```python
from build123d import *
from build123d.topology import SkipClean

# Parameters (mm, degrees)
EXTRUDE_1_DEPTH          = 80
SKETCH_2_R               = 13
CUT_EXTRUDE_2_DEPTH      = 15
CUT_EXTRUDE_START        = -15
SKETCH_4_R               = 13
CUT_EXTRUDE_3_DEPTH      = 15
CUT_EXTRUDE_4_DEPTH      = 123.918354375
CUT_EXTRUDE_4_DEPTH_BACK = 123.918354375
SKETCH_5_W               = 20
SKETCH_5_H               = 40
CUT_EXTRUDE_6_DEPTH      = 123.918354375
CUT_EXTRUDE_6_DEPTH_BACK = 24
CUT_EXTRUDE_7_DEPTH      = 131.345394404
CUT_EXTRUDE_8_DEPTH      = 32
CUT_EXTRUDE_8_DEPTH_BACK = 24
SKETCH_10_W              = 30
SKETCH_10_H              = 40
CUT_EXTRUDE_9_DEPTH      = 6
SKETCH_13_W              = 10.619852086
SKETCH_13_H              = 40
CUT_EXTRUDE_10_DEPTH     = 71
EXTRUDE_3_DEPTH          = 60


with BuildPart() as part:
    # Эскиз1 → Бобышка-Вытянуть1 (new body)
    with BuildSketch(Plane.XY):
        with BuildLine():
            Line((-84.314422505, -30), (-23.694570419, 25.759800711))
            ThreePointArc((-23.694570419, 25.759800711), (28.113366731, 20.847988178), (17.769230769, -30.153846154))
            Line((17.769230769, -30.153846154), (1.060606061, -40))
            Line((1.060606061, -40), (-84.314422505, -40))
            Line((-84.314422505, -40), (-84.314422505, -30))
        make_face()
    extrude(amount=EXTRUDE_1_DEPTH)

    # Эскиз2 → Вырез-Вытянуть2 (cut)
    with BuildSketch(Plane.XY):
        Circle(SKETCH_2_R)
    extrude(amount=CUT_EXTRUDE_2_DEPTH, mode=Mode.SUBTRACT)

    # Эскиз4 → Вырез-Вытянуть3 (cut)
    with BuildSketch(Plane.XY.offset(80).offset(CUT_EXTRUDE_START)):
        Circle(SKETCH_4_R)
    extrude(amount=CUT_EXTRUDE_3_DEPTH, mode=Mode.SUBTRACT)

    # Эскиз5 → Вырез-Вытянуть4 (cut, two sides: drawn at the far end of the back side and taken through both)
    with BuildSketch(Plane(origin=(0, 0, 0), x_dir=(1, 0, 0), z_dir=(0, 1, 0)).offset(-CUT_EXTRUDE_4_DEPTH_BACK)):
        with Locations((-74.314422505, -40)):
            Rectangle(SKETCH_5_W, SKETCH_5_H)
    extrude(amount=CUT_EXTRUDE_4_DEPTH + CUT_EXTRUDE_4_DEPTH_BACK, mode=Mode.SUBTRACT)

    # Эскиз6 → Вырез-Вытянуть6 (cut, two sides: drawn at the far end of the back side and taken through both)
    with BuildSketch(Plane(origin=(0, 0, 0), x_dir=(1, 0, 0), z_dir=(0, 1, 0)).offset(-CUT_EXTRUDE_6_DEPTH_BACK)):
        with BuildLine():
            Line((-55, -25), (-84.314422505, -25))
            Line((-84.314422505, -25), (-84.314422505, -55))
            Line((-84.314422505, -55), (-55, -55))
            ThreePointArc((-55, -55), (-40, -40), (-55, -25))
        make_face()
    extrude(amount=CUT_EXTRUDE_6_DEPTH + CUT_EXTRUDE_6_DEPTH_BACK, mode=Mode.SUBTRACT)

    # Эскиз9 → Вырез-Вытянуть7 (cut, through all)
    with BuildSketch(Plane(origin=(0, -24, 0), x_dir=(1, 0, 0), z_dir=(0, 1, 0))):
        with BuildLine():
            Line((-55, -48), (-92.733432528, -48))
            Line((-92.733432528, -48), (-92.733432528, -32))
            Line((-92.733432528, -32), (-55, -32))
            ThreePointArc((-55, -32), (-47, -40), (-55, -48))
        make_face()
    extrude(amount=-CUT_EXTRUDE_7_DEPTH, mode=Mode.SUBTRACT)

    # Эскиз10 → Вырез-Вытянуть8 (cut, two sides: drawn at the far end of the back side and taken through both)
    with BuildSketch(Plane(origin=(0, 0, 0), x_dir=(1, 0, 0), z_dir=(0, 1, 0)).offset(-CUT_EXTRUDE_8_DEPTH_BACK)):
        with Locations((-49.314422505, -40)):
            Rectangle(SKETCH_10_W, SKETCH_10_H)
    extrude(amount=CUT_EXTRUDE_8_DEPTH + CUT_EXTRUDE_8_DEPTH_BACK, mode=Mode.SUBTRACT)

    # Эскиз11 → Вырез-Вытянуть9 (cut)
    with BuildSketch(Plane(origin=(0, -24, 0), x_dir=(1, 0, 0), z_dir=(0, 1, 0))):
        with BuildLine():
            Line((-55, -25), (-81.861005174, -25))
            Line((-81.861005174, -25), (-81.861005174, -55))
            Line((-81.861005174, -55), (-55, -55))
            ThreePointArc((-55, -55), (-40, -40), (-55, -25))
        make_face()
    extrude(amount=-CUT_EXTRUDE_9_DEPTH, mode=Mode.SUBTRACT)

    # Эскиз13 → Вырез-Вытянуть10 (cut)
    with BuildSketch(Plane(origin=(0, -24, 0), x_dir=(1, 0, 0), z_dir=(0, 1, 0))):
        with Locations((-29.004496462, -40)):
            Rectangle(SKETCH_13_W, SKETCH_13_H)
    extrude(amount=CUT_EXTRUDE_10_DEPTH, mode=Mode.SUBTRACT)

    # Эскиз12 → Бобышка-Вытянуть3 (add)
    with SkipClean():  # the faces are left unmerged after this step: merging them gives an invalid solid
        with BuildSketch(Plane.XY):
            with BuildLine():
                Line((-35, 0), (-35, -24))
                Line((-35, -24), (-25.475478406, -24))
                ThreePointArc((-25.475478406, -24), (32.53184397, 12.9104271), (-35, 0))
            make_face()
        extrude(amount=EXTRUDE_3_DEPTH)


solid = part.part
```
Check sheet for the modelled part. Datum: model origin and axes. Units: mm. A direction names the side the tool comes from. Coordinates: 2 decimals unless noted, no trailing zeros. Order: outer loops, then holes, each group sorted by start corner. A loop starts at its lowest first (then second) coordinate and runs counter-clockwise, first axis right, second up. Notation, with made-up numbers: (34, 29.5) -> (62, 29.5) arc R34 cw to (62, 65.5) -> close; hole circle Ø6 at (73, 30). An arc over 180 degrees is marked (long way). Write each question's results on one line, items separated by ' | '. Start each with the question number.
1) Material ranges on line 1 along Z through (x, y) = (-50, -2); line 2 along Y through (x, z) = (0, 75.5); line 3 along Z through (x, y) = (5.5, -5), recorded low to high.
2) Section check D-D (z = 40). Enter the section's corners in (x, y).
3) Draft check along Z on faces 4 (the face through (-10.316, -7.91, 72.395)), 5 (the face through (0, 0, 65)), 6 (the face through (-60, -27, 25)), 7 (the face through (-60, -35, 32)). Enter one of: pulls with the +Z half, pulls with the -Z half, needs draft (parallel to the pull), parting line crosses it, or undercut.
4) Depth check by flat-ended pin: pin 1 (1.5 mm diameter, centred on y = -16, z = 63.5, fed in from -X); pin 2 (7 mm diameter, centred on y = -11.5, z = 38, fed in from -X); pin 3 (3.5 mm diameter, centred on y = -29.5, z = 56.5, fed in from -X). Enter the tip coordinate at first touch or a pass-through.
5) Section check C-C (y = 9). Enter the section's corners in (x, z), and give its area (3 significant figures).
6) Section check A-A (z = 67). Enter the section's corners in (x, y).
7) Section check B-B (x = -57.5). Enter the section's corners in (y, z), and give its area (3 significant figures).
8) Set-up check for faces 1 (the face through (-11, -10, 80)), 2 (the face through (-40, -27, 40)), 3 (the face through (-60, -35, 48)): record each of +Z, -Z, +X, -X, +Y, -Y from which the full face is reachable in a straight line by a thin tool's end or side.
Checked values:
1) line 1: 0 to 20, 60 to 80 | line 2: -40 to -13, 13 to 35 | line 3: 0 to 65
2) outline: (-47, -40) -> (1.06, -40) -> (17.77, -30.15) arc R35 ccw (long way) to (-35, 0) -> (-35, -24) -> (-40, -24) -> (-40, -30) -> (-47, -30) -> close
3) face 4: needs draft | face 5: pulls with the +Z half | face 6: undercut | face 7: undercut
4) pin 1: x = -69.91 | pin 2: x = -35 | pin 3: x = -64.31
5) outline: (-41.92, 0) -> (33.82, 0) -> (33.82, 80) -> (9.38, 80) -> (9.38, 65) -> (-9.38, 65) -> (-9.38, 80) -> (-41.92, 80) -> (-41.92, 60) -> (-33.82, 60) -> (-33.82, 20) -> (-41.92, 20) -> close | area: 5,450 mm²
6) outline: (-84.31, -40) -> (1.06, -40) -> (17.77, -30.15) arc R35 ccw (long way) to (-23.69, 25.76) -> (-84.31, -30) -> close; hole circle Ø26 at (0, 0)
7) outline: (-40, 0) -> (-5.34, 0) -> (-5.34, 20) -> (-24, 20) -> (-24, 25) -> (-30, 25) -> (-30, 32) -> (-40, 32) -> close; (-40, 48) -> (-30, 48) -> (-30, 55) -> (-24, 55) -> (-24, 60) -> (-5.34, 60) -> (-5.34, 80) -> (-40, 80) -> close | area: 1,690 mm²
8) face 1: +Z, +X, -X, +Y, -Y | face 2: -X, +Y | face 3: -X, +Y, -Y
